Geometry: final body of the model. Coordinates: model frame, mm. A direction names the side the tool comes from. Give positions to 0.01 mm unless a question says otherwise; leave off trailing zeros. Write each loop counter-clockwise with the first axis right and the second up, starting at its lowest first coordinate (ties: lowest second). Pieces come first, ordered by that corner, then holes.
```python
from build123d import *

# Parameters (mm, degrees)
ESQUISSE3_R                  = 3
ESQUISSE3_R_2                = 1.8
BOSS_EXTRU_1_DEPTH           = 1.4
ESQUISSE6_R                  = 2.25
ENL_V_MAT_EXTRU_2_DEPTH      = 1.8
ESQUISSE4_R                  = 5.15
ESQUISSE4_R_2                = 1.1
ENL_V_MAT_EXTRU_1_DEPTH      = 33.001953065
ENL_V_MAT_EXTRU_3_DEPTH      = 18.8
ENL_V_MAT_EXTRU_3_DEPTH_BACK = 18.8


with BuildPart() as part:
    # Esquisse2 → R_volution1 (revolve)
    with BuildSketch(Plane(origin=(0, 0, 0), x_dir=(0, 0, -1), z_dir=(1, 0, 0)), mode=Mode.PRIVATE) as r_volution1_sk:
        Polygon((0, 0), (0, 17.4), (-12.3, 18.783814786), (-12.3, 21.126244206), (-13.4, 21.25), (-13.4, 17.7), (-2.4, 16.462442061), (-2.4, 0), align=None)
    revolve(r_volution1_sk.sketch.rotate(Axis((0, 0, 0), (0, 0, 1)), 90), axis=Axis((0, 0, 0), (0, 0, 1)))

    # Esquisse3 → Boss.-Extru.1 (add)
    # profile 1 of 4: a face of its own
    with BuildSketch(Plane(origin=(0, 0, 0), x_dir=(-1, 0, 0), z_dir=(0, 0, -1))):
        with Locations((0, -8.199894223)):
            Circle(ESQUISSE3_R)
        with Locations((0, -8.199894223)):
            Circle(ESQUISSE3_R_2, mode=Mode.SUBTRACT)
    # profile 2 of 4: a face of its own
    with BuildSketch(Plane(origin=(0, 0, 0), x_dir=(-1, 0, 0), z_dir=(0, 0, -1))):
        with Locations((-8.199894223, 0)):
            Circle(ESQUISSE3_R)
        with Locations((-8.199894223, 0)):
            Circle(ESQUISSE3_R_2, mode=Mode.SUBTRACT)
    # profile 3 of 4: a face of its own
    with BuildSketch(Plane(origin=(0, 0, 0), x_dir=(-1, 0, 0), z_dir=(0, 0, -1))):
        with Locations((0, 8.199894223)):
            Circle(ESQUISSE3_R)
        with Locations((0, 8.199894223)):
            Circle(ESQUISSE3_R_2, mode=Mode.SUBTRACT)
    # profile 4 of 4: a face of its own
    with BuildSketch(Plane(origin=(0, 0, 0), x_dir=(-1, 0, 0), z_dir=(0, 0, -1))):
        with Locations((8.199894223, 0)):
            Circle(ESQUISSE3_R)
        with Locations((8.199894223, 0)):
            Circle(ESQUISSE3_R_2, mode=Mode.SUBTRACT)
    extrude(amount=BOSS_EXTRU_1_DEPTH)

    # Esquisse6 → Enl_v. mat.-Extru.2 (cut)
    with BuildSketch(Plane.XY.offset(2.4)):
        with Locations((0, 8.199894223)):
            Circle(ESQUISSE6_R)
        with Locations((8.199894223, 0)):
            Circle(ESQUISSE6_R)
        with Locations((0, -8.199894223)):
            Circle(ESQUISSE6_R)
        with Locations((-8.199894223, 0)):
            Circle(ESQUISSE6_R)
    extrude(amount=-ENL_V_MAT_EXTRU_2_DEPTH, mode=Mode.SUBTRACT)

    # Esquisse4 → Enl_v. mat.-Extru.1 (cut, through all)
    with BuildSketch(Plane.XY.offset(2.4)):
        Circle(ESQUISSE4_R)
        with Locations((0, 8.199894223)):
            Circle(ESQUISSE4_R_2)
        with Locations((8.199894223, 0)):
            Circle(ESQUISSE4_R_2)
        with Locations((0, -8.199894223)):
            Circle(ESQUISSE4_R_2)
        with Locations((-8.199894223, 0)):
            Circle(ESQUISSE4_R_2)
    extrude(amount=-ENL_V_MAT_EXTRU_1_DEPTH, mode=Mode.SUBTRACT)

    # Esquisse7 → Enl_v. mat.-Extru.3 (cut, two sides: drawn at the far end of the back side and taken through both)
    with BuildSketch(Plane(origin=(0, 0, 0), x_dir=(0, 0, -1), z_dir=(1, 0, 0)).offset(-ENL_V_MAT_EXTRU_3_DEPTH_BACK)):
        with BuildLine():
            Line((-13.4, 1.55), (-6.827902443, 1.44983161))
            ThreePointArc((-6.827902443, 1.44983161), (-5.4, 0), (-6.827902443, -1.44983161))
            Line((-6.827902443, -1.44983161), (-13.4, -1.55))
            Line((-13.4, -1.55), (-13.4, 1.55))
        make_face()
    extrude(amount=ENL_V_MAT_EXTRU_3_DEPTH + ENL_V_MAT_EXTRU_3_DEPTH_BACK, mode=Mode.SUBTRACT)


solid = part.part
```
Item 1: Pin query (flat end, axial travel): pin 1 Ø5 at (y, z) = (6.5, 1) entering from -X; pin 2 Ø3 at (x, y) = (-8.2, 0) entering from +Z; pin 3 Ø4 at (x, y) = (-8.2, 0) entering from -Z; pin 4 Ø6 at (y, z) = (-5.5, 2) entering from -X. Return the tip coordinate at first contact, or that it passes through.
Found:
pin 1: stops at x = -17.12
pin 2: stops at z = 0.6
pin 3: stops at z = -1.4
pin 4: stops at x = -17.56
Item 2: Pull-direction query (Y, two-part tool) for faces 5 (the face through (10, 0, -1)), 6 (the face through (5.43, -1.15, -0.69)); classes: +Y half, -Y half, draft (parallel to the pull), parting line (faces both ways), or undercut.
Found:
face 5: undercut
face 6: parting line
Item 3: Section D-D, the plane z = 1.25. Return the cut outline in (x, y).
Found:
outline: circle Ø35.08 at (0, 0); hole circle Ø4.5 at (-8.2, 0); hole circle Ø10.3 at (0, 0); hole circle Ø4.5 at (0, -8.2); hole circle Ø4.5 at (0, 8.2); hole circle Ø4.5 at (8.2, 0)
Item 4: Reachability of faces 1 (the face through (-1, 7, 0.6)), 2 (the face through (0.391, 11.174, -0.69)), 3 (the face through (-18.8, 0, 13)), 4 (the face through (17.4, 0, 5.4)) from +Z, -Z, +X, -X, +Y, -Y: full face, straight path, thin tool, end or side. Return the list, or none.
Found:
face 1: +Z
face 2: -Z
face 3: +Z, -Z
face 4: +Z, +X, -X
Item 5: Line query: L1, parallel to Y at x = 0, z = -0.75; L2, parallel to Z at x = -5.5, y = -9; L3, parallel to X at y = -12, z = 6.75. Output: solid intervals per line, ascending.
Found:
L1: y = -11.2 to -10, -6.4 to -5.2, 5.2 to 6.4, 10 to 11.2
L2: z = 0 to 2.4
L3: x = -13.63 to -11.97, 11.97 to 13.63
Item 6: Section B-B, the plane x = 0. State how many separate pieces and enclosed holes the cut face has, plus the area to 3 significant figures.
Found:
separate pieces: 4
enclosed holes: 0
area: 79.0 mm2
